Study the drawing (mm; zero at the part's minimum x, y, z) and answer. A direction names the side the tool comes from. Round coordinates to 2 decimals unless told otherwise and drop trailing zeros. Loops run counter-clockwise (first coordinate to the right, second up) from the corner with the lowest first, then second, coordinate; pieces in that order, holes last. Notation, with made-up numbers: (46.5, 55) -> (58.5, 55) arc R26 cw to (58.5, 82) -> close; hole circle Ø7 at (3, 57). An arc over 180 degrees is marked (long way). Use one line per item in the form item = value.
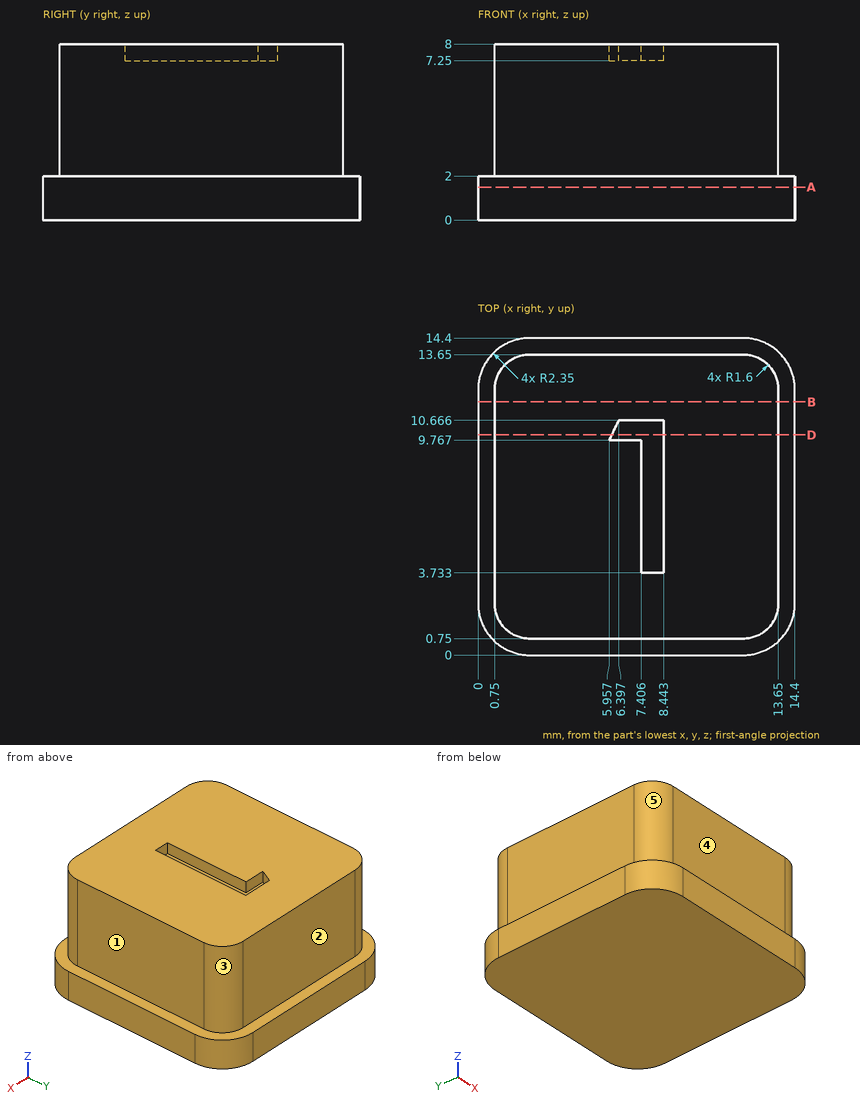
(1) Consider L1, parallel to X at y = 4.25, z = 6; L2, parallel to X at y = 1, z = 1 (1 decimal). Determine where each line is inside the solid, lowest interval first.
Completed:
L1 = 0.75 to 13.65
L2 = 0.4 to 14
(2) For the marked faces 1, 2, 3, 4 and 5, determine the directions among +Z, -Z, +X, -X, +Y, -Y from which every point of the face is accessible in a straight line to the end or side of a thin tool.
Completed:
face_1 = +Z, +X, +Y, -Y
face_2 = +Z, +X, -X, +Y
face_3 = +Z, +X, +Y
face_4 = +Z, +X, -X, -Y
face_5 = +Z, -X, -Y
(3) Find section A-A, the plane z = 1.5. Write down the section's boundary in (x, y), then the cut area to 3 significant figures.
Completed:
outline = (0, 2.35) arc R2.35 ccw to (2.35, 0) -> (12.05, 0) arc R2.35 ccw to (14.4, 2.35) -> (14.4, 12.05) arc R2.35 ccw to (12.05, 14.4) -> (2.35, 14.4) arc R2.35 ccw to (0, 12.05) -> close
area = 203 mm2
(4) Find section D-D, the plane y = 10. Write down the section's boundary in (x, z), then the cut area to 3 significant figures.
Completed:
outline = (0, 0) -> (14.4, 0) -> (14.4, 2) -> (13.65, 2) -> (13.65, 8) -> (8.44, 8) -> (8.44, 7.25) -> (6.07, 7.25) -> (6.07, 8) -> (0.75, 8) -> (0.75, 2) -> (0, 2) -> close
area = 104 mm2
(5) Find section B-B, the plane y = 11.5. Write down the section's boundary in (x, z).
Completed:
outline = (0, 0) -> (14.4, 0) -> (14.4, 2) -> (13.65, 2) -> (13.65, 8) -> (0.75, 8) -> (0.75, 2) -> (0, 2) -> close
(6) Given P1, Ø0.6, axis at y = 7, z = 7.5, coming from the -X side; P2, Ø3, axis at x = 9, z = 5.5, coming from the +Y side; P3, Ø0.6, axis at y = 6.5, z = 7.5, coming from the +X side, each flat-ended and moving along its own axis, determine where each tip first touches the part or whether it passes through.
Completed:
P1 = 0.75
P2 = 13.65
P3 = 13.65
